Input: part model. Units: mm. Frame: model coordinates. A direction names the side the tool comes from. Give positions to 0.01 mm unless a question says otherwise; leave off trailing zeros. Loops run counter-clockwise (first coordinate to the right, second up) from the corner with the lowest first, then second, coordinate; pieces in that order, holes last.
from build123d import *

# Parameters (mm, degrees)
SKETCH1_R               = 16
BOSS_EXTRUDE1_DEPTH     = 40
SKETCH2_R               = 11.2
CUT_EXTRUDE1_DEPTH      = 46.956501172
SKETCH3_OUTSIDE_W       = 46.08
SKETCH3_OUTSIDE_H       = 46.08
SKETCH3_OUTSIDE_R       = 13.5
CUT_EXTRUDE2_DEPTH      = 35
CUT_EXTRUDE3_START      = -3
CUT_EXTRUDE3_DEPTH      = 3
CUT_EXTRUDE9_DEPTH      = 46.956501172
CUT_EXTRUDE9_DEPTH_BACK = 3
BOSS_EXTRUDE3_START     = -1.5
BOSS_EXTRUDE3_DEPTH     = 1.5
BOSS_EXTRUDE4_START     = 5
BOSS_EXTRUDE4_DEPTH     = 5
CUT_EXTRUDE10_START     = 3
CUT_EXTRUDE10_DEPTH     = 3
CUT_EXTRUDE11_DEPTH     = 3
BOSS_EXTRUDE5_DEPTH     = 1.5
CUT_EXTRUDE12_DEPTH     = 46.956501172
CUT_EXTRUDE13_DEPTH     = 1


with BuildPart() as part:
    # Sketch1 → Boss-Extrude1 (new body)
    with BuildSketch(Plane(origin=(0, 0, 0), x_dir=(0, 0, -1), z_dir=(1, 0, 0))):
        Circle(SKETCH1_R)
    extrude(amount=BOSS_EXTRUDE1_DEPTH)

    # Sketch2 → Cut-Extrude1 (cut, through all)
    with BuildSketch(Plane(origin=(40, 0, 0), x_dir=(0, 0, -1), z_dir=(1, 0, 0))):
        Circle(SKETCH2_R)
    extrude(amount=-CUT_EXTRUDE1_DEPTH, mode=Mode.SUBTRACT)

    # Sketch3 outside → Cut-Extrude2 (cut)
    with BuildSketch(Plane(origin=(40, 0, 0), x_dir=(0, 0, -1), z_dir=(1, 0, 0))):
        Rectangle(SKETCH3_OUTSIDE_W, SKETCH3_OUTSIDE_H)
        Circle(SKETCH3_OUTSIDE_R, mode=Mode.SUBTRACT)
    extrude(amount=-CUT_EXTRUDE2_DEPTH, mode=Mode.SUBTRACT)

    # Sketch4 → Cut-Extrude3 (cut)
    with BuildSketch(Plane.ZY.offset(CUT_EXTRUDE3_START)):
        with BuildLine():
            Line((-4, 10.461357464), (-4, 13.461357464))
            ThreePointArc((-4, 13.461357464), (0, 14.043081741), (4, 13.461357464))
            Line((4, 13.461357464), (4, 10.461357464))
            ThreePointArc((4, 10.461357464), (0, 11.2), (-4, 10.461357464))
        make_face()
    extrude(amount=CUT_EXTRUDE3_DEPTH, mode=Mode.SUBTRACT)

    # Sketch11 → Cut-Extrude9 (cut, two sides: drawn at the far end of the back side and taken through both)
    with BuildSketch(Plane.ZY.offset(-CUT_EXTRUDE9_DEPTH_BACK)):
        with BuildLine():
            Line((31.521155816, -96.172447268), (4.983269846, -15.204177769))
            Line((4.983269846, -15.204177769), (4, -12.204177769))
            ThreePointArc((4, -12.204177769), (0, -12.842972982), (-4, -12.204177769))
            Line((-4, -12.204177769), (-4.983269846, -15.204177769))
            Line((-4.983269846, -15.204177769), (-31.521155816, -96.172447268))
            Line((-31.521155816, -96.172447268), (-31.521155816, -266.585123526))
            Line((-31.521155816, -266.585123526), (31.521155816, -266.585123526))
            Line((31.521155816, -266.585123526), (31.521155816, -96.172447268))
        make_face()
    extrude(amount=CUT_EXTRUDE9_DEPTH + CUT_EXTRUDE9_DEPTH_BACK, mode=Mode.SUBTRACT)

    # Sketch15 → Boss-Extrude3 (add)
    with BuildSketch(Plane.ZY.offset(BOSS_EXTRUDE3_START)):
        with BuildLine():
            Line((-4, -12.204177769), (-4.327756615, -13.204177769))
            ThreePointArc((-4.327756615, -13.204177769), (0, -13.895315322), (4.327756615, -13.204177769))
            Line((4.327756615, -13.204177769), (4, -12.204177769))
            ThreePointArc((4, -12.204177769), (0, -12.842972982), (-4, -12.204177769))
        make_face()
        with BuildLine():
            Line((-4, 12.461357464), (-4, 13.461357464))
            ThreePointArc((-4, 13.461357464), (0, 14.043081741), (4, 13.461357464))
            Line((4, 13.461357464), (4, 12.461357464))
            ThreePointArc((4, 12.461357464), (0, 13.087605964), (-4, 12.461357464))
        make_face()
    extrude(amount=BOSS_EXTRUDE3_DEPTH)

    # Sketch16 → Boss-Extrude4 (add)
    with BuildSketch(Plane(origin=(40, 0, 0), x_dir=(0, 0, -1), z_dir=(1, 0, 0)).offset(BOSS_EXTRUDE4_START)):
        with BuildLine():
            Line((-4, 10.461357464), (-4, 13.461357464))
            ThreePointArc((-4, 13.461357464), (0, 14.043081741), (4, 13.461357464))
            Line((4, 13.461357464), (4, 10.461357464))
            ThreePointArc((4, 10.461357464), (0, 11.2), (-4, 10.461357464))
        make_face()
        with BuildLine():
            Line((-4, -10.461357464), (-5.357142857, -14.010746604))
            ThreePointArc((-5.357142857, -14.010746604), (0, -15), (5.357142857, -14.010746604))
            Line((5.357142857, -14.010746604), (4, -10.461357464))
            ThreePointArc((4, -10.461357464), (0, -11.2), (-4, -10.461357464))
        make_face()
    extrude(amount=-BOSS_EXTRUDE4_DEPTH)

    # Sketch17 → Cut-Extrude10 (cut)
    with BuildSketch(Plane(origin=(40, 0, 0), x_dir=(0, 0, -1), z_dir=(1, 0, 0)).offset(CUT_EXTRUDE10_START)):
        with BuildLine():
            Line((-4, 13.461357464), (-4, 12.461357464))
            ThreePointArc((-4, 12.461357464), (0, 13.087605964), (4, 12.461357464))
            Line((4, 12.461357464), (4, 13.461357464))
            ThreePointArc((4, 13.461357464), (0, 14.043081741), (-4, 13.461357464))
        make_face()
    extrude(amount=-CUT_EXTRUDE10_DEPTH, mode=Mode.SUBTRACT)

    # Sketch18 → Cut-Extrude11 (cut)
    with BuildSketch(Plane(origin=(45, 0, 0), x_dir=(0, 0, -1), z_dir=(1, 0, 0))):
        with BuildLine():
            Line((-4, -10.461357464), (-4.714285714, -12.329457012))
            ThreePointArc((-4.714285714, -12.329457012), (0, -13.2), (4.714285714, -12.329457012))
            Line((4.714285714, -12.329457012), (4, -10.461357464))
            ThreePointArc((4, -10.461357464), (0, -11.2), (-4, -10.461357464))
        make_face()
    extrude(amount=-CUT_EXTRUDE11_DEPTH, mode=Mode.SUBTRACT)

    # Sketch21 → Boss-Extrude5 (add)
    with BuildSketch(Plane(origin=(45, 0, 0), x_dir=(0, 0, -1), z_dir=(1, 0, 0))):
        with BuildLine():
            Line((-4.714285714, -12.329457012), (-4.357142857, -11.395407238))
            ThreePointArc((-4.357142857, -11.395407238), (0, -12.2), (4.357142857, -11.395407238))
            Line((4.357142857, -11.395407238), (4.714285714, -12.329457012))
            ThreePointArc((4.714285714, -12.329457012), (0, -13.2), (-4.714285714, -12.329457012))
        make_face()
    extrude(amount=-BOSS_EXTRUDE5_DEPTH)

    # Sketch22 → Cut-Extrude12 (cut, through all)
    with BuildSketch(Plane(origin=(40, 0, 0), x_dir=(0, 0, -1), z_dir=(1, 0, 0))):
        with BuildLine():
            Line((7.673498409, -9.029962065), (8.430853573, -8.376958883))
            ThreePointArc((8.430853573, -8.376958883), (9.136032746, -8.429134874), (9.083856755, -9.134314047))
            Line((9.083856755, -9.134314047), (8.326501591, -9.787317229))
            ThreePointArc((8.326501591, -9.787317229), (7.621322418, -9.735141237), (7.673498409, -9.029962065))
        make_face()
        with BuildLine():
            Line((-9.134721879, -9.238785274), (-9.806253772, -8.497809622))
            ThreePointArc((-9.806253772, -8.497809622), (-9.771531893, -7.79155585), (-9.065278121, -7.826277729))
            Line((-9.065278121, -7.826277729), (-8.393746228, -8.567253381))
            ThreePointArc((-8.393746228, -8.567253381), (-8.428468107, -9.273507153), (-9.134721879, -9.238785274))
        make_face()
    extrude(amount=-CUT_EXTRUDE12_DEPTH, mode=Mode.SUBTRACT)

    # Sketch23 → Cut-Extrude13 (cut)
    with BuildSketch(Plane.ZY):
        with BuildLine():
            Line((9.771531893, -7.79155585), (10.985476817, -8.672656141))
            ThreePointArc((10.985476817, -8.672656141), (0.600129097, -13.983401249), (-10.202038674, -9.581965994))
            Line((-10.202038674, -9.581965994), (-9.136032746, -8.429134874))
            Line((-9.136032746, -8.429134874), (-7.502618183, -9.357538492))
            ThreePointArc((-7.502618183, -9.357538492), (0.59553752, -11.979070969), (8.393746228, -8.567253381))
            Line((8.393746228, -8.567253381), (9.771531893, -7.79155585))
        make_face()
    extrude(amount=-CUT_EXTRUDE13_DEPTH, mode=Mode.SUBTRACT)


solid = part.part
(1) Cut plane D-D (y = 5). Return the cut outline in (x, z).
Values follow:
outline: (0, -15.2) - (5, -15.2) - (5, -12.54) - (40, -12.54) - (40, -10.02) - (0, -10.02) - close; (0, 10.02) - (40, 10.02) - (40, 12.54) - (5, 12.54) - (5, 15.2) - (0, 15.2) - close
(2) Pin query (flat end, axial travel): pin 1 Ø10 at (x, y) = (22.5, 10) entering from -Z; pin 2 Ø3.5 at (x, y) = (43.5, 12) entering from +Z; pin 3 Ø0.9 at (x, y) = (1.5, 11.5) entering from -Z. Return the tip coordinate at first contact, or that it passes through.
Values follow:
pin 1: stops at z = -12.54
pin 2: stops at z = 4
pin 3: stops at z = -11.57
(3) Cut plane B-B (x = 39). Return the cut outline in (y, z).
Values follow:
outline: circle Ø27 at (0, 0); hole circle Ø22.4 at (0, 0); hole (-9.79, -8.33) - (-9.13, -9.08) arc R0.5 ccw to (-8.38, -8.43) - (-9.03, -7.67) arc R0.5 ccw to start; hole (-9.24, 9.13) arc R0.5 ccw to (-8.57, 8.39) - (-7.83, 9.07) arc R0.5 ccw to (-8.5, 9.81) - close
(4) Reachability of faces 4 (the cylindrical face through (44.014, 14.043, 0.057)), 5 (the flat face through (3, -14, 0)), 6 (the flat face through (1, -12.2, 0.5)), 7 (the flat face through (43, 12, -4)), 8 (the flat face through (1.5, 13.4, 0.1)) from +Z, -Z, +X, -X, +Y, -Y: full face, straight path, thin tool, end or side. Return the list, or none.
Values follow:
face 4: +X, +Y
face 5: -Y
face 6: -X
face 7: -Z, +X, +Y
face 8: none
(5) Ray query, probe 1 along Z at (x, y) = (9, 0); probe 2 along X at (y, z) = (-14, -1.5). Return the intervals inside material, ascending.
Values follow:
probe 1: z = -13.5 to -11.2, 11.2 to 13.5
probe 2: x = 3 to 5, 40 to 45
(6) Mould query, pull axis Y, two halves, no side actions, for faces 1 (the cylindrical face through (2.26, 14.043, -0.057)), 2 (the flat face through (1.5, -13, 0)), 3 (the cylindrical face through (41.521, 13.087, 0.057)). Classes: +Y half, -Y half, draft (parallel to the pull), parting line (faces both ways), or undercut.
Values follow:
face 1: undercut
face 2: draft
face 3: +Y half
(7) Cut plane C-C (y = 0). Return the cut outline in (x, z), and give its area (3 significant figures).
Values follow:
outline: (0, -16) - (5, -16) - (5, -13.5) - (40, -13.5) - (40, -11.2) - (0, -11.2) - close; (0, 11.2) - (40, 11.2) - (40, 13.5) - (5, 13.5) - (5, 16) - (0, 16) - close
area: 209 mm2
